Read the model definition and answer for the solid it produces. Units are mm, in the model's axes. A direction names the side the tool comes from. Coordinates: 2 decimals unless noted, no trailing zeros. Write each loop counter-clockwise with the first axis right and the second up, starting at its lowest first coordinate (ties: lowest second). Pieces come first, ordered by that corner, then holes. Notation, with made-up numbers: (73.25, -17) -> (122.25, -17) arc R17 cw to (122.25, 8) -> close; hole circle Ø11 at (7.5, -5). An arc over 180 degrees is marked (long way). Answer as a JSON object with one key per item and string values. Group by question number.
(1) Which of the six approach directions +Z, -Z, +X, -X, +Y, -Y give full straight-line access (tool end or side, diameter ignored) to faces 5 (the face through (-2.1, 0.66, 4.36)), 6 (the face through (0, 0, 0))?
(2) Flat-ended cylindrical pins translate along their axes: P1, Ø1.5, axis at x = -0.5, y = 0.5, coming from the +Z side; P2, Ø2, axis at y = -4, z = 2.5, coming from the +X side; P3, Ø5, axis at x = -1, y = -0.5, coming from the +Z side; P4, Ø1, axis at y = 2.5, z = 2.5, coming from the -X side. Find the tip coordinate at first contact, or state that the pin passes through.
(3) For a pull along Y with two mould halves and no side action, classify faces 1 (the face through (-2.1, 0.66, 1.86)), 2 (the face through (3.3, 0.1, 1)), 3 (the face through (0.585, -2.636, 2.878)), 4 (the face through (0, 0, 1.3)) as +Y half, -Y half, draft (parallel to the pull), parting line (faces both ways), or undercut.
(4) Straight lines are drawn through the part: L1, parallel to Y at x = 0, z = 4.15; L2, parallel to Z at x = -0.25, y = 3.5; L3, parallel to Z at x = 1.25, y = 1. For each, find the intervals that lie inside material, in ascending order.
(5) Find section C-C (z = 4.05). Give the vertices of the cut face in (x, y).
from build123d import *

# Parameters (mm, degrees)
F0_W = 2.2
F0_H = 0.3
F2_R = 0.49999
F3_R = 0.3


# Not quite as in the source:
# - a fillet or chamfer is up to 0.001 mm smaller than in the source, because OpenCascade refuses the exact size


with BuildPart() as f1:
    # F0 (on Front) → F1 (revolve)
    with BuildSketch(Plane.XZ):
        Polygon((-2.7, 1), (-5, 1), (-5, 0), (0, 0), (0, 1), (-2.2, 1), align=None)
        Polygon((-2.7, 5), (-2.7, 1), (-2.2, 1), (-2.2, 1.3), (-2.2, 2.4), (-2.2, 3.7), (-2.2, 5), align=None)
        with BuildLine():
            Line((-2.2, 3.7), (-2.2, 2.4))
            ThreePointArc((-2.2, 2.4), (-1.55, 3.05), (-2.2, 3.7))
        make_face()
        with Locations((-1.1, 1.15)):
            Rectangle(F0_W, F0_H)
    revolve(axis=Axis((0, 0, 0.5), (0, 0, -1)))

    # F2 (radius 0.5 in the source; OpenCascade refuses exactly that, so slightly less here)
    f2_edges = [f1.edges().sort_by_distance(p)[0] for p in [
        (2.7, 0, 5),
        (5, 0, 0),
    ]]
    fillet(f2_edges, radius=F2_R)

    # F3
    f3_edges = [f1.edges().sort_by_distance(p)[0] for p in [
        (2.7, 0, 1),
    ]]
    fillet(f3_edges, radius=F3_R)


solid = f1.part
Results below:
{
 "1": {"face 5": "+Z", "face 6": "-Z, +X, -X, +Y, -Y"},
 "2": {"P1": "stops at z = 1.3", "P2": "passes through", "P3": "stops at z = 5", "P4": "stops at x = -1.81"},
 "3": {"face 1": "undercut", "face 2": "draft", "face 3": "parting line", "face 4": "undercut"},
 "4": {"L1": "y = -2.7 to -2.2, 2.2 to 2.7", "L2": "z = 0 to 1", "L3": "z = 0 to 1.3, 2.8 to 3.3"},
 "5": {"outline": "circle Ø5.4 at (0, 0); hole circle Ø4.4 at (0, 0)"}
}
